Autodesk Inventor part; units mm, degrees
ref_plane "Work Plane1" through (-17.4436, 0, 0) normal (0, -0.866, -0.5) x (1, 0, 0)
ref_plane "YZ Plane" through (0, 0, 0) normal (1, 0, 0) x (0, 1, 0)
ref_plane "XZ Plane" through (0, 0, 0) normal (0, 1, 0) x (-1, 0, 0)
sketch "Эскиз1" plane through (0, 0, 0) normal (1, 0, 0) x (0, 1, 0)
  line L0 (-9.2376, 0) -> (-4.6188, 8)
  line L1 (-4.6188, 8) -> (4.6188, 8)
  line L2 (4.6188, 8) -> (9.2376, 0)
  line L3 (9.2376, 0) -> (4.6188, -8)
  line L4 (4.6188, -8) -> (-4.6188, -8)
  line L5 (-4.6188, -8) -> (-9.2376, 0)
  point P0 (0, 0)
  point P1 (0, 0)
  dimension "d0" = 18.4752
extrude "Базовый элемент" add sketch "Эскиз1" along normal blind 8.4
sketch "Эскиз2" plane through (0, 0, 0) normal (0, 0, 1) x (1, 0, 0)
  line L0 (0, 4.6188) -> (0, 9.2376)
  line L1 (0, 9.2376) -> (8.4, 9.2376)
  line L2 (8.4, 4.6188) -> (8.4, 9.2376)
  line L3 (-1.68, 0) -> (10.08, 0)
  line L4 (0.5771, 9.2376) -> (0, 8)
  line L5 (7.8229, 9.2376) -> (8.4, 8)
  dimension "d3" = 25
  dimension "d4" = 25
  dimension "d5" = 16
  dimension "d6" = 16
revolve "Фаска1" cut sketch "Эскиз2" angle 360 about axis through (-10, 0, 0) along (1, 0, 0)
sketch "Эскиз3" plane through (8.4, 0, 0) normal (1, 0, 0) x (0, 0, -1)
  arc A0 (-4, -6.9282) -> (4, -6.9282) centre (0, 0) ccw
hole "Резьба" at (8.4, 0, 0) direction (-1, 0, 0) diameter 8.376 end through all
chamfer "Фаска2" distance 0.8119 angle 30 1 edges at (8.4, 0, 4.188) measured on face at (8.4, 6.6899, -0.1683)
chamfer "Фаска3" distance 0.8119 angle 30 1 edges at (0, 0, 4.188) measured on face at (0, 6.6899, -0.1683)
ref_plane "Work Plane1" through (-17.4436, 0, 0) normal (0, -0.866, -0.5) x (1, 0, 0)
equation "\"d0\" = 1.1547 * SW"
equation "\"d1\" = KOH"
equation "\"d3\" = ANG1"
equation "\"d4\" = ANG2"
equation "\"d5\" = SW0"
equation "\"d6\" = SW01"
equation "\"d8\" = -0.5 * GD1 + 0.5 * NND"
equation "\"d40\" = -0.5 * GD1 + 0.5 * NND"
equation "\"d10\" = -0.5 * GD1 + 0.5 * NND"
equation "\"d41\" = -0.5 * GD1 + 0.5 * NND"
equation "\"ANG1\" = 25deg"
equation "\"ANG2\" = 25deg"
equation "\"KOH\" = 8.4"
equation "\"SW\" = 16"
equation "\"SW0\" = SW"
equation "\"SW01\" = SW"
equation "\"GUL\" = 0.541266 * PTC"
equation "\"TOA\" = 30deg"
equation "\"PTC\" = 1.5"
equation "\"E0\" = 1.155 * SW"
equation "\"GAL\" = 0.541266 * PTC"
equation "\"SD2\" = 0"
equation "\"WFT\" = 0"
properties part number "ANSI B 18.2.4.1 M - M10 x 1,5" material "Сталь, мягкая"
Can you work these out from the model? Positions are in its coordinate system, mm. Give positions to 0.01 mm unless a question says otherwise; leave off trailing zeros. Order: outer loops, then holes, each group sorted by start corner. A loop starts at its lowest first (then second) coordinate and runs counter-clockwise, first axis right, second up. Notation, with made-up numbers: M -12.75,69 L 34.25,69 A23 ccw 34.25,80 Z; hole C -21,76 d9. An arc over 180 degrees is marked long. Write item = value, one per line. Start each with the question number.
Q1. Will these pins go through, and if not, where does the flat tip stop? pin 1 Ø1.5 at (x, z) = (5.5, -5.5) entering from -Y; pin 2 Ø1.5 at (y, z) = (-3.5, 0.5) entering from +X; pin 3 Ø9.5 at (y, z) = (0, 0) entering from -X.
Q2. We'd pull the mould along Z, two halves only. Please class faces 1 (the conical face through (8.26, 8.3, 0.02)), 2 (the cylindrical face through (4.148, -2.83, 3.087)), 3 (the conical face through (8.26, -4.17, 7.18)), 4 (the flat face through (4, 0, -8)): pulls with the +Z half, pulls with the -Z half, needs draft (parallel to the pull), parting line crosses it, or undercut.
Q3. I need wall thicknesses on probe 1 along Z at (x, y) = (3.5, 0); probe 2 along Z at (x, y) = (7.75, 3.5); probe 3 along Y at (x, z) = (7, 2.5). Which ranges of each line are inside material? Lowest first, please. Write a range as [from, to].
Q4. Suppose I cut it at A-A (x = 4.75). Write out the boundary of the cut face in (y, z).
Check result:
q1.pin_1 = -6.5
q1.pin_2 = 7.99
q1.pin_3 = 0.14
q2.face_1 = parting line crosses it
q2.face_2 = undercut
q2.face_3 = pulls with the +Z half
q2.face_4 = pulls with the -Z half
q3.probe_1 = [-8, -4.19], [4.19, 8]
q3.probe_2 = [-8, -2.3], [2.3, 8]
q3.probe_3 = [-7.79, -3.36], [3.36, 7.79]
q4.outline = M -9.24,0 L -4.62,-8 L 4.62,-8 L 9.24,0 L 4.62,8 L -4.62,8 Z; hole C 0,0 d8.38
